Here's how the part is built. I have some questions about the finished solid (model axes, mm). Face numbers are marked on the shaded views. Coordinates: 2 decimals unless noted, no trailing zeros. Write each loop counter-clockwise with the first axis right and the second up, starting at its lowest first coordinate (ties: lowest second). Pieces come first, ordered by that corner, then holes. Notation, with made-up numbers: (65.25, 52.5) -> (96.25, 52.5) arc R17 cw to (96.25, 57.5) -> close; hole circle Ø5 at (15.25, 42.25). An arc over 180 degrees is marked (long way). Use a Markdown table: item, result. Add a question column.
Item 1: Will these pins go through, and if not, where does the flat tip stop? pin 1 Ø6 at (x, z) = (10, 10.5) entering from +Y; pin 2 Ø2 at (x, z) = (-10.5, 6.5) entering from +Y; pin 3 Ø14.5 at (x, z) = (-1, -2) entering from -Y.
Item 2: Imagine slicing it at A-A, the plane y = 37. Write out the boundary of the cut face in (x, z), and give its area (3 significant figures).
Item 3: If we mould it in two halves opening along Z, with no side actions, what happens to the marked faces 1 and 2? For each: pulls with the +Z half, pulls with the -Z half, needs draft (parallel to the pull), parting line crosses it, or undercut.
Item 4: If I drill on line 1 along Z through (x, y) = (0, 2); line 2 along X through (y, z) = (37.5, 0); line 3 along Y through (x, z) = (-6.5, 9), over which ranges is the centre line in solid material (lowest first)? Write a range as from..to.
Autodesk Inventor part; units mm, degrees
ref_plane "YZ Plane" through (0, 0, 0) normal (1, 0, 0) x (0, 1, 0)
ref_plane "XZ Plane" through (0, 0, 0) normal (0, 1, 0) x (-1, 0, 0)
ref_plane "XY Plane" through (0, 0, 0) normal (0, 0, 1) x (1, 0, 0)
sketch "Sketch1" plane through (0, 0, 0) normal (0, 1, 0) x (-1, 0, 0)
  circle A0 centre (0, 0) radius 22.5
  circle A1 centre (0, 0) radius 19.5
  circle A2 centre (0, 0) radius 12.7
  circle A3 centre (0, 0) radius 6
  circle A4 centre (8.8049, 3.6331) radius 1.63
  circle A5 centre (7.5488, -5.8087) radius 1.63
  circle A6 centre (-1.2561, -9.4418) radius 1.63
  circle A7 centre (-8.8049, -3.6331) radius 1.63
  circle A8 centre (-7.5488, 5.8087) radius 1.63
  circle A9 centre (1.2561, 9.4418) radius 1.63
  circle A10 centre (0, 0) radius 14.7
  dimension "d0" = 45
  dimension "d1" = 3
  dimension "d4" = 2
extrude "Extrusion1" add sketch "Sketch1" along normal blind 4 contours A1
sketch "Sketch2" plane through (0, 4, 0) normal (0, 1, 0) x (1, 0, 0)
  circle A0 centre (0, 0) radius 19.5
  circle A1 centre (0, 0) radius 14.7
  circle A2 centre (-7.5488, 5.8087) radius 1.63
  circle A3 centre (-8.8049, -3.6331) radius 1.63
  circle A4 centre (-1.2561, -9.4418) radius 1.63
  circle A5 centre (7.5488, -5.8087) radius 1.63
  circle A6 centre (8.8049, 3.6331) radius 1.63
  circle A7 centre (1.2561, 9.4418) radius 1.63
  circle A8 centre (0, 0) radius 12.7
extrude "Extrusion2" add sketch "Sketch2" along normal blind 2 contours A0 | A1 | A8
sketch "Sketch3" plane through (0, 6, 0) normal (0, 1, 0) x (1, 0, 0)
  circle A0 centre (0, 0) radius 22.5
  circle A1 centre (0, 0) radius 19.5
  circle A2 centre (0, 0) radius 18.5
  dimension "d7" = 45
  dimension "d8" = 3
  dimension "d9" = 1
extrude "Extrusion3" add sketch "Sketch3" along normal blind 47 contours A1
fillet "Fillet1" radius 2 1 edges at (-18.5, 6, 0)
properties part number "tulejka"
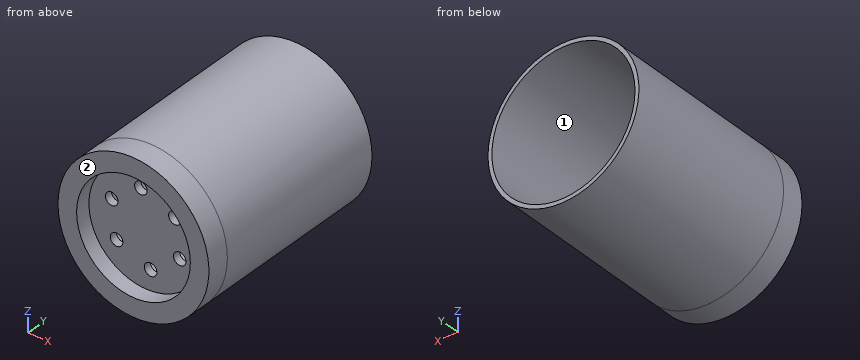
Ans:
| question | item | result |
|---|---|---|
| 1 | pin 1 | stops at y = 6.27 |
| 1 | pin 2 | stops at y = 6 |
| 1 | pin 3 | stops at y = 4 |
| 2 | outline | circle Ø39 at (0, 0); hole circle Ø37 at (0, 0) |
| 2 | area | 119 mm^2 |
| 3 | face 1 | undercut |
| 3 | face 2 | needs draft |
| 4 | line 1 | z = -19.5..-14.7, 14.7..19.5 |
| 4 | line 2 | x = -19.5..-18.5, 18.5..19.5 |
| 4 | line 3 | y = 4..6 |
